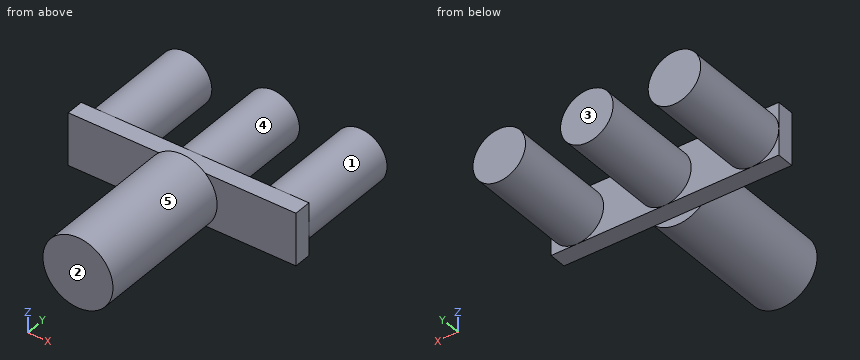
from build123d import *

# Parameters (mm, degrees)
F0_W     = 65
F0_H     = 15
F1_DEPTH = 5
F2_R     = 7.5
F3_DEPTH = 30
F4_R     = 10
F5_DEPTH = 40


with BuildPart() as f1:
    # F0 (on Front) → F1 (new body)
    with BuildSketch(Plane.XZ):
        Rectangle(F0_W, F0_H)
    extrude(amount=F1_DEPTH)

    # F2 (on face) → F3 (join)
    with BuildSketch(Plane(origin=(0, 0, 0), x_dir=(-1, 0, 0), z_dir=(0, 1, 0))):
        with BuildLine():
            ThreePointArc((-7.5, 0), (0, -7.5), (7.5, 0))
            ThreePointArc((7.5, 0), (0, 7.5), (-7.5, 0))
        make_face()
        with Locations((-25, 0)):
            Circle(F2_R)
        with BuildLine():
            ThreePointArc((32.5, 0), (25, 7.5), (17.5, 0))
            ThreePointArc((17.5, 0), (25, -7.5), (32.5, 0))
        make_face()
    extrude(amount=F3_DEPTH)

    # F4 (on face) → F5 (join)
    with BuildSketch(Plane.XZ.offset(5)):
        Circle(F4_R)
    extrude(amount=F5_DEPTH)


solid = f1.part
Read the model definition and answer for the solid it produces. Units are mm, in the model's axes. Face numbers are marked on the shaded views. A direction names the side the tool comes from. Coordinates: 2 decimals unless noted, no trailing zeros. Write each loop counter-clockwise with the first axis right and the second up, starting at its lowest first coordinate (ties: lowest second). Pieces come first, ordered by that corner, then holes. Notation, with made-up numbers: M 84.25,16.5 L 124.25,16.5 A26 ccw 124.25,53.5 Z; hole C 46,26.25 d2. An arc over 180 degrees is marked long. Use a Markdown table: item, result.
Q1. The part is cut by section C-C, the plane y = -10. Write down the section's boundary in (x, z), then the cut area to 3 significant figures.
Answer block:
| item | result |
|---|---|
| outline | C 0,0 d20 |
| area | 314 mm2 |
Q2. Determine the mould class of the marked faces 3, 4 and 5 for opening direction X: released by +X, released by -X, zero draft, split by the parting line, or undercut.
Answer block:
| item | result |
|---|---|
| face 3 | zero draft |
| face 4 | undercut |
| face 5 | split by the parting line |
Q3. Each of these flat-tipped pins is pushed along its axis until it touches: pin 1 Ø3 at (x, y) = (-6, 3.5) entering from -Z; pin 2 Ø1 at (x, z) = (18, -7) entering from -Y; pin 3 Ø5.5 at (x, y) = (13, -3.5) entering from +Z. Where does it stop, or does it pass through?
Answer block:
| item | result |
|---|---|
| pin 1 | stops at z = -6 |
| pin 2 | stops at y = -5 |
| pin 3 | stops at z = 7.5 |
Q4. The part is cut by section D-D, the plane x = -12.5. Write down the section's boundary in (y, z).
Answer block:
| item | result |
|---|---|
| outline | M -5,-7.5 L 0,-7.5 L 0,7.5 L -5,7.5 Z |
Q5. The part is cut by section B-B, the plane y = 17.5. Write down the section's boundary in (x, z), then the cut area to 3 significant figures.
Answer block:
| item | result |
|---|---|
| outline | C -25,0 d15; C 0,0 d15; C 25,0 d15 |
| area | 530 mm2 |
Q6. Which of the six approach directions +Z, -Z, +X, -X, +Y, -Y give full straight-line access (tool end or side, diameter ignored) to the marked faces 1 and 2?
Answer block:
| item | result |
|---|---|
| face 1 | +Y |
| face 2 | +Z, -Z, +X, -X, -Y |
Q7. Straight lines are drawn through the part: L1, parallel to X at y = 20, z = 0.5; L2, parallel to Y at x = 17, z = 1; L3, parallel to X at y = 18, z = 5.25. For each, find the intervals that lie inside material, in ascending order. Write a range as [from, to].
Answer block:
| item | result |
|---|---|
| L1 | x = [-32.48, -17.52], [-7.48, 7.48], [17.52, 32.48] |
| L2 | y = [-5, 0] |
| L3 | x = [-30.36, -19.64], [-5.36, 5.36], [19.64, 30.36] |
Q8. The part is cut by section A-A, the plane x = -1. Write down the section's boundary in (y, z), then the cut area to 3 significant figures.
Answer block:
| item | result |
|---|---|
| outline | M -45,-9.95 L -5,-9.95 L -5,-7.5 L 0,-7.5 L 0,-7.43 L 30,-7.43 L 30,7.43 L 0,7.43 L 0,7.5 L -5,7.5 L -5,9.95 L -45,9.95 Z |
| area | 1,320 mm2 |
